Geometry: final body of the model. Coordinates: model frame, mm. Face numbers are marked on the shaded views. Give positions to 0.01 mm unless a question says otherwise; leave off trailing zeros. Order: outer loops, then holes, each group sorted by start corner. A loop starts at its lowest first (then second) coordinate and runs counter-clockwise, first axis right, second up. Notation, with made-up numbers: (-33.5, 14.25) - (-20.5, 14.25) arc R26 cw to (-20.5, 42.25) - close; hole circle Ø6 at (13.25, 68.5). An arc over 180 degrees is marked (long way). One line per item, written item: value.
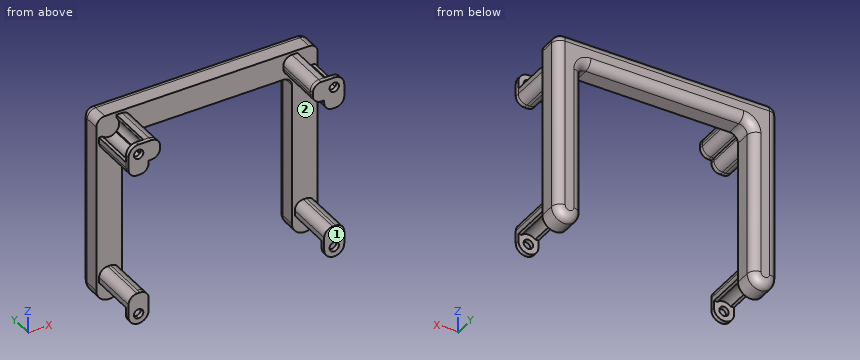
```python
from build123d import *

# Parameters (mm, degrees)
SKETCH1_R             = 2.9718
SKETCH1_R_2           = 1.397
BOSS_EXTRUDE1_DEPTH   = 1.27
BOSS_EXTRUDE1_2_DEPTH = 1.27
BOSS_EXTRUDE1_3_DEPTH = 1.27
BOSS_EXTRUDE1_4_DEPTH = 1.27
BOSS_EXTRUDE2_DEPTH   = 6.985
FILLET1_R             = 2.54
BOSS_EXTRUDE3_DEPTH   = 1.27
BOSS_EXTRUDE4_DEPTH   = 13.081


with BuildPart() as part:
    # Sketch1 → Boss-Extrude1 (new body)
    with BuildSketch(Plane(origin=(0, 0, 0), x_dir=(1, 0, 0), z_dir=(0, 1, 0))):
        with Locations(Location((0, 0, 0), (0, 0, 270))):
            Circle(SKETCH1_R)
        with Locations(Location((0, 0, 0), (0, 0, 270))):
            Circle(SKETCH1_R_2, mode=Mode.SUBTRACT)
    extrude(amount=BOSS_EXTRUDE1_DEPTH)



with BuildPart() as body_2:
    # Sketch1 → Boss-Extrude1 2 (new body)
    with BuildSketch(Plane(origin=(0, 0, 0), x_dir=(1, 0, 0), z_dir=(0, 1, 0))):
        with Locations(Location((58.039, 0, 0), (0, 0, 90))):
            Circle(SKETCH1_R)
        with Locations(Location((58.039, 0, 0), (0, 0, 90))):
            Circle(SKETCH1_R_2, mode=Mode.SUBTRACT)
    extrude(amount=BOSS_EXTRUDE1_2_DEPTH)


with BuildPart() as body_3:
    # Sketch1 → Boss-Extrude1 3 (new body)
    with BuildSketch(Plane(origin=(0, 0, 0), x_dir=(1, 0, 0), z_dir=(0, 1, 0))):
        with Locations(Location((58.039, 48.895, 0), (0, 0, 270))):
            Circle(SKETCH1_R)
        with Locations(Location((58.039, 48.895, 0), (0, 0, 270))):
            Circle(SKETCH1_R_2, mode=Mode.SUBTRACT)
    extrude(amount=BOSS_EXTRUDE1_3_DEPTH)


with BuildPart() as body_4:
    # Sketch1 → Boss-Extrude1 4 (new body)
    with BuildSketch(Plane(origin=(0, 0, 0), x_dir=(1, 0, 0), z_dir=(0, 1, 0))):
        with Locations(Location((0, 48.895, 0), (0, 0, 90))):
            Circle(SKETCH1_R)
        with Locations(Location((0, 48.895, 0), (0, 0, 90))):
            Circle(SKETCH1_R_2, mode=Mode.SUBTRACT)
    extrude(amount=BOSS_EXTRUDE1_4_DEPTH)


with BuildPart() as body_5:
    # Sketch2 → Boss-Extrude2 (new body)
    with BuildSketch(Plane(origin=(0, 14.351, 0), x_dir=(1, 0, 0), z_dir=(0, 1, 0))):
        with BuildLine():
            Line((-3.81, 48.895), (-3.81, -1.27))
            ThreePointArc((-3.81, -1.27), (-3.066051224, -3.066051224), (-1.27, -3.81))
            Line((-1.27, -3.81), (59.309, -3.81))
            ThreePointArc((59.309, -3.81), (61.105051224, -3.066051224), (61.849, -1.27))
            Line((61.849, -1.27), (61.849, 48.895))
            ThreePointArc((61.849, 48.895), (58.039, 52.705), (54.229, 48.895))
            Line((54.229, 48.895), (54.229, 6.35))
            ThreePointArc((54.229, 6.35), (53.485051224, 4.553948776), (51.689, 3.81))
            Line((51.689, 3.81), (6.35, 3.81))
            ThreePointArc((6.35, 3.81), (4.553948776, 4.553948776), (3.81, 6.35))
            Line((3.81, 6.35), (3.81, 48.895))
            ThreePointArc((3.81, 48.895), (0, 52.705), (-3.81, 48.895))
        make_face()
    extrude(amount=BOSS_EXTRUDE2_DEPTH)

    # Fillet1
    fillet1_edges = [body_5.edges().sort_by_distance(p)[0] for p in [
        (-3.066051224, 21.336, 3.066051224),
        (29.0195, 21.336, 3.81),
        (61.105051224, 21.336, 3.066051224),
        (61.849, 21.336, -23.8125),
        (58.039, 21.336, -52.705),
        (54.229, 21.336, -27.6225),
        (53.485051224, 21.336, -4.553948776),
        (29.0195, 21.336, -3.81),
        (4.553948776, 21.336, -4.553948776),
        (3.81, 21.336, -27.6225),
        (0, 21.336, -52.705),
        (-3.81, 21.336, -23.8125),
    ]]
    fillet(fillet1_edges, radius=FILLET1_R)


with BuildPart() as part_1:
    add(part.part)

    add(body_2.part)  # Boss-Extrude3 merges body 2

    add(body_3.part)  # Boss-Extrude3 merges body 3

    add(body_4.part)  # Boss-Extrude3 merges body 4
    # Sketch3 → Boss-Extrude3 (add)
    with BuildSketch(Plane.XZ):
        with BuildLine():
            Line((-1.397, -48.895), (-2.9718, -48.895))
            Line((-2.9718, -48.895), (-2.9718, -45.085))
            ThreePointArc((-2.9718, -45.085), (-2.227851224, -43.288948776), (-0.4318, -42.545))
            Line((-0.4318, -42.545), (0.4318, -42.545))
            ThreePointArc((0.4318, -42.545), (2.227851224, -43.288948776), (2.9718, -45.085))
            Line((2.9718, -45.085), (2.9718, -48.895))
            Line((2.9718, -48.895), (1.397, -48.895))
            ThreePointArc((1.397, -48.895), (0, -47.498), (-1.397, -48.895))
        make_face()
        with BuildLine():
            Line((-2.9718, -3.81), (-2.9718, 0))
            Line((-2.9718, 0), (-1.397, 0))
            ThreePointArc((-1.397, 0), (0.987828173, -0.987828173), (0, 1.397))
            Line((0, 1.397), (0, 2.9718))
            Line((0, 2.9718), (3.81, 2.9718))
            ThreePointArc((3.81, 2.9718), (5.606051224, 2.227851224), (6.35, 0.4318))
            Line((6.35, 0.4318), (6.35, -0.4318))
            ThreePointArc((6.35, -0.4318), (5.606051224, -2.227851224), (3.81, -2.9718))
            Line((3.81, -2.9718), (2.9718, -2.9718))
            Line((2.9718, -2.9718), (2.9718, -3.81))
            ThreePointArc((2.9718, -3.81), (2.227851224, -5.606051224), (0.4318, -6.35))
            Line((0.4318, -6.35), (-0.4318, -6.35))
            ThreePointArc((-0.4318, -6.35), (-2.227851224, -5.606051224), (-2.9718, -3.81))
        make_face()
        with BuildLine():
            Line((59.436, 0), (61.0108, 0))
            Line((61.0108, 0), (61.0108, -3.81))
            ThreePointArc((61.0108, -3.81), (60.266851224, -5.606051224), (58.4708, -6.35))
            Line((58.4708, -6.35), (57.6072, -6.35))
            ThreePointArc((57.6072, -6.35), (55.811148776, -5.606051224), (55.0672, -3.81))
            Line((55.0672, -3.81), (55.0672, -2.9718))
            Line((55.0672, -2.9718), (54.229, -2.9718))
            ThreePointArc((54.229, -2.9718), (52.432948776, -2.227851224), (51.689, -0.4318))
            Line((51.689, -0.4318), (51.689, 0.4318))
            ThreePointArc((51.689, 0.4318), (52.432948776, 2.227851224), (54.229, 2.9718))
            Line((54.229, 2.9718), (58.039, 2.9718))
            Line((58.039, 2.9718), (58.039, 1.397))
            ThreePointArc((58.039, 1.397), (57.051171827, -0.987828173), (59.436, 0))
        make_face()
        with BuildLine():
            Line((61.0108, -45.085), (61.0108, -48.895))
            Line((61.0108, -48.895), (59.436, -48.895))
            ThreePointArc((59.436, -48.895), (58.039, -47.498), (56.642, -48.895))
            Line((56.642, -48.895), (55.0672, -48.895))
            Line((55.0672, -48.895), (55.0672, -45.085))
            ThreePointArc((55.0672, -45.085), (55.811148776, -43.288948776), (57.6072, -42.545))
            Line((57.6072, -42.545), (58.4708, -42.545))
            ThreePointArc((58.4708, -42.545), (60.266851224, -43.288948776), (61.0108, -45.085))
        make_face()
    extrude(amount=-BOSS_EXTRUDE3_DEPTH)


    add(body_5.part)  # Boss-Extrude4 merges body 5
    # Sketch4 → Boss-Extrude4 (add)
    with BuildSketch(Plane(origin=(0, 1.27, 0), x_dir=(1, 0, 0), z_dir=(0, 1, 0))):
        with BuildLine():
            Line((-2.9718, 46.7106), (-2.014942153, 46.7106))
            ThreePointArc((-2.014942153, 46.7106), (0, 45.9232), (2.014942153, 46.7106))
            Line((2.014942153, 46.7106), (2.9718, 46.7106))
            Line((2.9718, 46.7106), (2.9718, 45.085))
            ThreePointArc((2.9718, 45.085), (2.227851224, 43.288948776), (0.4318, 42.545))
            Line((0.4318, 42.545), (-0.4318, 42.545))
            ThreePointArc((-0.4318, 42.545), (-2.227851224, 43.288948776), (-2.9718, 45.085))
            Line((-2.9718, 45.085), (-2.9718, 46.7106))
        make_face()
        with BuildLine():
            Line((56.024057847, 46.7106), (55.0672, 46.7106))
            Line((55.0672, 46.7106), (55.0672, 45.085))
            ThreePointArc((55.0672, 45.085), (55.811148776, 43.288948776), (57.6072, 42.545))
            Line((57.6072, 42.545), (58.4708, 42.545))
            ThreePointArc((58.4708, 42.545), (60.266851224, 43.288948776), (61.0108, 45.085))
            Line((61.0108, 45.085), (61.0108, 46.7106))
            Line((61.0108, 46.7106), (60.053942153, 46.7106))
            ThreePointArc((60.053942153, 46.7106), (58.039, 45.9232), (56.024057847, 46.7106))
        make_face()
        with BuildLine():
            Line((2.014942153, 2.1844), (2.1844, 2.1844))
            Line((2.1844, 2.1844), (2.1844, 2.014942153))
            ThreePointArc((2.1844, 2.014942153), (2.9718, 0), (2.1844, -2.014942153))
            Line((2.1844, -2.014942153), (2.1844, -2.9718))
            Line((2.1844, -2.9718), (3.81, -2.9718))
            ThreePointArc((3.81, -2.9718), (5.606051224, -2.227851224), (6.35, -0.4318))
            Line((6.35, -0.4318), (6.35, 0.4318))
            ThreePointArc((6.35, 0.4318), (5.606051224, 2.227851224), (3.81, 2.9718))
            Line((3.81, 2.9718), (2.9718, 2.9718))
            Line((2.9718, 2.9718), (2.9718, 3.81))
            ThreePointArc((2.9718, 3.81), (2.227851224, 5.606051224), (0.4318, 6.35))
            Line((0.4318, 6.35), (-0.4318, 6.35))
            ThreePointArc((-0.4318, 6.35), (-2.227851224, 5.606051224), (-2.9718, 3.81))
            Line((-2.9718, 3.81), (-2.9718, 2.1844))
            Line((-2.9718, 2.1844), (-2.014942153, 2.1844))
            ThreePointArc((-2.014942153, 2.1844), (0, 2.9718), (2.014942153, 2.1844))
        make_face()
        with BuildLine():
            Line((55.8546, 2.014942153), (55.8546, 2.1844))
            Line((55.8546, 2.1844), (56.024057847, 2.1844))
            ThreePointArc((56.024057847, 2.1844), (58.039, 2.9718), (60.053942153, 2.1844))
            Line((60.053942153, 2.1844), (61.0108, 2.1844))
            Line((61.0108, 2.1844), (61.0108, 3.81))
            ThreePointArc((61.0108, 3.81), (60.266851224, 5.606051224), (58.4708, 6.35))
            Line((58.4708, 6.35), (57.6072, 6.35))
            ThreePointArc((57.6072, 6.35), (55.811148776, 5.606051224), (55.0672, 3.81))
            Line((55.0672, 3.81), (55.0672, 2.9718))
            Line((55.0672, 2.9718), (54.229, 2.9718))
            ThreePointArc((54.229, 2.9718), (52.432948776, 2.227851224), (51.689, 0.4318))
            Line((51.689, 0.4318), (51.689, -0.4318))
            ThreePointArc((51.689, -0.4318), (52.432948776, -2.227851224), (54.229, -2.9718))
            Line((54.229, -2.9718), (55.8546, -2.9718))
            Line((55.8546, -2.9718), (55.8546, -2.014942153))
            ThreePointArc((55.8546, -2.014942153), (55.0672, 0), (55.8546, 2.014942153))
        make_face()
    extrude(amount=BOSS_EXTRUDE4_DEPTH)


solid = part_1.part
```
1) Material intervals for line 1 along X through (y, z) = (0.3, 0); line 2 along X through (y, z) = (10.25, -3.5); line 3 along X through (y, z) = (16.5, -39), sorted ascending.
Answers below:
line 1: -2.97 to -1.4, 1.4 to 6.35, 51.69 to 56.64, 59.44 to 61.01
line 2: -2.97 to 2.97, 55.07 to 61.01
line 3: -3.81 to 3.81, 54.23 to 61.85
2) Section B-B, the plane y = 7. Count the separate pieces of the cut face and the enclosed holes in it, then the cut area to 3 significant figures.
Answers below:
separate pieces: 4
enclosed holes: 0
area: 118 mm^2
3) Section A-A, the plane z = -28. Return loops of the section in (x, y), then the cut area to 3 significant figures.
Answers below:
outline: (-3.81, 14.35) - (3.81, 14.35) - (3.81, 18.8) arc R2.54 ccw to (1.27, 21.34) - (-1.27, 21.34) arc R2.54 ccw to (-3.81, 18.8) - close; (54.23, 14.35) - (61.85, 14.35) - (61.85, 18.8) arc R2.54 ccw to (59.31, 21.34) - (56.77, 21.34) arc R2.54 ccw to (54.23, 18.8) - close
area: 101 mm^2
4) Section C-C, the plane x = 19. Return loops of the section in (y, z), then the cut area to 3 significant figures.
Answers below:
outline: (14.35, -3.81) - (18.8, -3.81) arc R2.54 ccw to (21.34, -1.27) - (21.34, 1.27) arc R2.54 ccw to (18.8, 3.81) - (14.35, 3.81) - close
area: 50.5 mm^2
5) First-contact query: pin 1 (0.8 mm diameter, centred on x = 55.5, y = 8.5, fed in from +Z); pin 2 (6 mm diameter, centred on x = 8.5, z = -2.5, fed in from -Y); pin 3 (0.7 mm diameter, centred on y = 0.5, z = -3.5, fed in from -X); pin 4 (3 mm diameter, centred on x = 50, y = 9.5, fed in from -Z). Flat tips, straight axial feed; report the tip coordinate or a pass-through.
Answers below:
pin 1: z = 2.97
pin 2: y = 0
pin 3: x = -2.97
pin 4: through
6) Mould query, pull axis X, two halves, no side actions, for the marked faces 1 and 2. Classes: released by +X, released by -X, zero draft, split by the parting line, or undercut.
Answers below:
face 1: zero draft
face 2: undercut
